The listing builds one solid part. Answer for the finished solid, in the listing's coordinates (mm). Face numbers are marked on the shaded views. A direction names the side the tool comes from. Round coordinates to 2 decimals unless told otherwise and drop trailing zeros. Write each loop counter-clockwise with the first axis right and the second up, starting at its lowest first coordinate (ties: lowest second). Pieces come first, ordered by that corner, then holes.
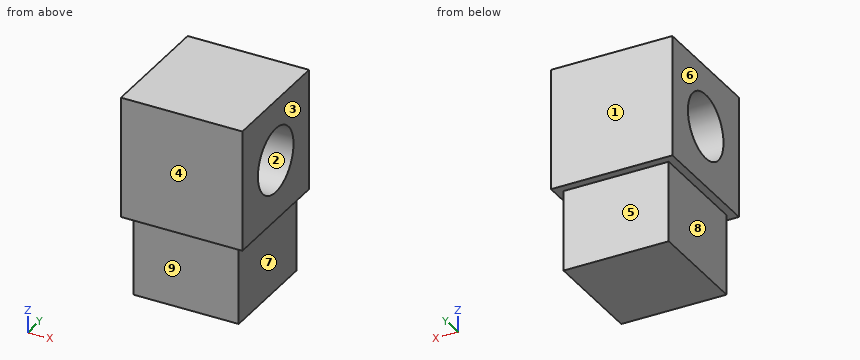
from build123d import *

# Parameters (mm, degrees)
F0_W     = 13
F0_H     = 13
F1_DEPTH = 10
F2_W     = 15
F2_H     = 15
F2_W_2   = 13
F2_H_2   = 13
F3_DEPTH = 15
F4_R     = 4
F5_DEPTH = 25


with BuildPart() as f1:
    # F0 (on Top) → F1 (new body)
    with BuildSketch(Plane.XY):
        Rectangle(F0_W, F0_H)
    extrude(amount=F1_DEPTH)

    # F2 (on face) → F3 (join)
    with BuildSketch(Plane.XY.offset(10)):
        Rectangle(F2_W, F2_H)
        Rectangle(F2_W_2, F2_H_2, mode=Mode.SUBTRACT)
        Rectangle(F2_W_2, F2_H_2)
    extrude(amount=F3_DEPTH)

    # F4 (on face) → F5 (cut)
    with BuildSketch(Plane.YZ.offset(7.5)):
        with Locations((0, 17.5)):
            Circle(F4_R)
    extrude(amount=-F5_DEPTH, mode=Mode.SUBTRACT)


solid = f1.part
1. For a pull along Y with two mould halves and no side action, classify the marked faces 1, 2, 3 and 4 as released by +Y, released by -Y, zero draft, split by the parting line, or undercut.
Geometry says:
face 1: released by +Y
face 2: undercut
face 3: zero draft
face 4: released by -Y
2. Section D-D on y = 5.25 is taken. Determine the outline of the cut face in (x, z), plus the area to 3 significant figures.
Geometry says:
outline: (-7.5, 10) - (-6.5, 10) - (-6.5, 0) - (6.5, 0) - (6.5, 10) - (7.5, 10) - (7.5, 25) - (-7.5, 25) - close
area: 355 mm2
3. A tool of negligible diameter and unlimited length cuts with its end or side. For the marked faces 5, 6, 7, 8 and 9, from which of +Z, -Z, +X, -X, +Y, -Y can it reach the whole face along a straight path? Write none if from no direction.
Geometry says:
face 5: -Z, +X, -X, +Y
face 6: +Z, -Z, -X, +Y, -Y
face 7: -Z, +X, +Y, -Y
face 8: -Z, -X, +Y, -Y
face 9: -Z, +X, -X, -Y
4. Section B-B on z = 17.5 is taken. Determine the outline of the cut face in (x, y), plus the area to 3 significant figures.
Geometry says:
outline: (-7.5, -7.5) - (7.5, -7.5) - (7.5, -4) - (-7.5, -4) - close; (-7.5, 4) - (7.5, 4) - (7.5, 7.5) - (-7.5, 7.5) - close
area: 105 mm2
5. Section C-C on x = 1 is taken. Determine the outline of the cut face in (y, z), plus the area to 3 significant figures.
Geometry says:
outline: (-7.5, 10) - (-6.5, 10) - (-6.5, 0) - (6.5, 0) - (6.5, 10) - (7.5, 10) - (7.5, 25) - (-7.5, 25) - close; hole circle Ø8 at (0, 17.5)
area: 305 mm2
6. Given pin 1 (5 mm diameter, centred on y = 0, z = 17.5, fed in from -X); pin 2 (3 mm diameter, centred on y = 3, z = 6.5, fed in from +X); pin 3 (6 mm diameter, centred on x = 3, z = 5, fed in from -Y); pin 4 (5 mm diameter, centred on x = 2.5, z = 6.5, fed in from +Y), each flat-ended and moving along its own axis, determine where each tip first touches the part or whether it passes through.
Geometry says:
pin 1: passes through
pin 2: stops at x = 6.5
pin 3: stops at y = -6.5
pin 4: stops at y = 6.5
7. Section A-A on y = 0 is taken. Determine the outline of the cut face in (x, z).
Geometry says:
outline: (-7.5, 10) - (-6.5, 10) - (-6.5, 0) - (6.5, 0) - (6.5, 10) - (7.5, 10) - (7.5, 13.5) - (-7.5, 13.5) - close; (-7.5, 21.5) - (7.5, 21.5) - (7.5, 25) - (-7.5, 25) - close
8. Straight lines are drawn through the part: line 1 along Z through (x, y) = (-1.5, 0); line 2 along X through (y, z) = (0, 8.75); line 3 along Z through (x, y) = (4.75, -3.5). For each, find the intervals that lie inside material, in ascending order.
Geometry says:
line 1: z = 0 to 13.5, 21.5 to 25
line 2: x = -6.5 to 6.5
line 3: z = 0 to 15.56, 19.44 to 25
